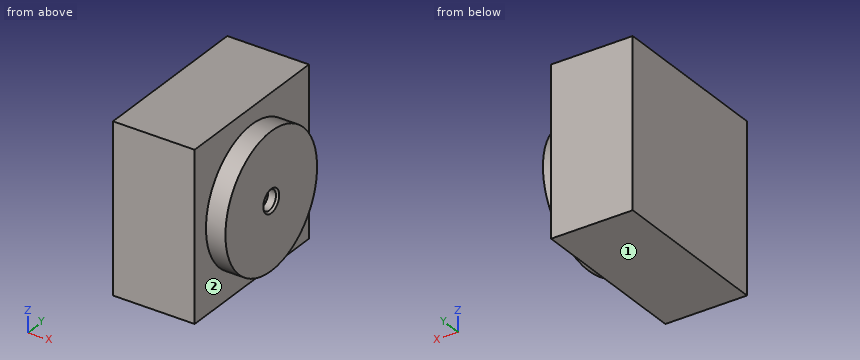
Autodesk Inventor part; units mm, degrees
ref_plane "YZ Plane" through (0, 0, 0) normal (1, 0, 0) x (0, 1, 0)
ref_plane "XZ Plane" through (0, 0, 0) normal (0, 1, 0) x (-1, 0, 0)
ref_plane "XY Plane" through (0, 0, 0) normal (0, 0, 1) x (1, 0, 0)
sketch "스케치1" plane through (0, 0, 0) normal (1, 0, 0) x (0, 1, 0)
  line L0 (4.3, 4.3) -> (-4.3, 4.3)
  line L1 (-4.3, 4.3) -> (-4.3, -4.3)
  line L2 (-4.3, -4.3) -> (4.3, -4.3)
  line L3 (4.3, -4.3) -> (4.3, 4.3)
  line L4 (4.3, 4.3) -> (-4.3, -4.3) construction
  line L5 (-4.3, 4.3) -> (4.3, -4.3) construction
  point P0 (0, 0)
  dimension "d0" = 8.6
  dimension "d1" = 8.6
extrude "돌출1" add sketch "스케치1" along normal blind 4.2
sketch "스케치2" plane through (4.2, 0, 0) normal (1, 0, 0) x (0, 0, -1)
  circle A0 centre (0, 0) radius 3.45
  dimension "d4" = 6.9
extrude "돌출2" add sketch "스케치2" along normal blind 1
sketch "스케치3" plane through (5.2, 0, 0) normal (1, 0, 0) x (0, 0, -1)
  circle A0 centre (0, 0) radius 0.5
  dimension "d7" = 1
extrude "돌출3" cut sketch "스케치3" against normal blind 0.5
chamfer "모따기1" distance 0.1 angle 45 1 edges at (5.2, 0, 0.5)
properties part number "카메라"
Here's how the part is built. I have some questions about the finished solid (model axes, mm). Face numbers are marked on the shaded views. A direction names the side the tool comes from. Give positions to 0.01 mm unless a question says otherwise; leave off trailing zeros. Loops run counter-clockwise (first coordinate to the right, second up) from the corner with the lowest first, then second, coordinate; pieces in that order, holes last. Notation, with made-up numbers: (27.5, 61.5) -> (48.5, 61.5) arc R20 ccw to (48.5, 71.5) -> close; hole circle Ø9 at (9, -26). An arc over 180 degrees is marked (long way). One line per item, written item: value.
Q1. On a 3-axis mill with a long thin cutter (end or side, diameter ignored), from which of +Z, -Z, +X, -X, +Y, -Y can I reach the whole of each face in a straight line? I mean the marked faces 1 and 2. Say none if no direction works.
Answers follow:
face 1: -Z, +X, -X, +Y, -Y
face 2: +X
Q2. If I drill on line 1 along Y through (x, z) = (4.8, 0); line 2 along X through (y, z) = (0.5, -3.5); line 3 along Y through (x, z) = (4.95, -0.25), over which ranges is the centre line in solid material (lowest first)?
Answers follow:
line 1: -3.45 to -0.5, 0.5 to 3.45
line 2: 0 to 4.2
line 3: -3.44 to -0.43, 0.43 to 3.44
Q3. Suppose I cut it at D-D on z = -2. Please give me the cut outline in (x, y), then the cut area to 3 significant figures.
Answers follow:
outline: (0, -4.3) -> (4.2, -4.3) -> (4.2, -2.81) -> (5.2, -2.81) -> (5.2, 2.81) -> (4.2, 2.81) -> (4.2, 4.3) -> (0, 4.3) -> close
area: 41.7 mm^2
Q4. Suppose I cut it at A-A on y = 0. Please give me the cut outline in (x, z), then the cut area to 3 significant figures.
Answers follow:
outline: (0, -4.3) -> (4.2, -4.3) -> (4.2, -3.45) -> (5.2, -3.45) -> (5.2, -0.6) -> (5.1, -0.5) -> (4.7, -0.5) -> (4.7, 0.5) -> (5.1, 0.5) -> (5.2, 0.6) -> (5.2, 3.45) -> (4.2, 3.45) -> (4.2, 4.3) -> (0, 4.3) -> close
area: 42.5 mm^2
Q5. Suppose I cut it at C-C on y = 1.5. Please give me the cut outline in (x, z), then the cut area to 3 significant figures.
Answers follow:
outline: (0, -4.3) -> (4.2, -4.3) -> (4.2, -3.11) -> (5.2, -3.11) -> (5.2, 3.11) -> (4.2, 3.11) -> (4.2, 4.3) -> (0, 4.3) -> close
area: 42.3 mm^2
